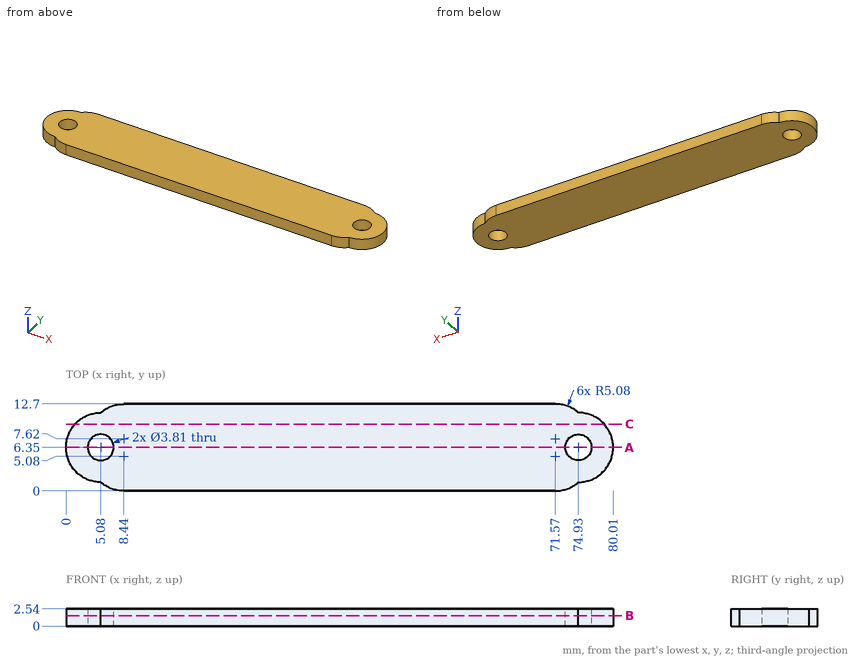
Here's the drawing with two shaded views (mm, measured from the low corner). I have some questions. Coordinates: 2 decimals unless noted, no trailing zeros. Order: outer loops, then holes, each group sorted by start corner. A loop starts at its lowest first (then second) coordinate and runs counter-clockwise, first axis right, second up. Notation, with made-up numbers: (-29.75, 80.5) - (27.25, 80.5) arc R15 cw to (27.25, 94.5) - close; hole circle Ø4 at (-19.5, -19.75). An arc over 180 degrees is marked (long way). Use CSV: the item, a comma, the result in double quotes. Start each with the question number.
1. Suppose I cut it at A-A on y = 6.35. List the corners of the cut face in (x, z) for me (3 decimals), then the cut area to 3 significant figures.
2. I'm going to push flat-ended pins straight in: pin 1 (1 mm diameter, centred on y = 9, z = 1.5, fed in from +X); pin 2 (2.5 mm diameter, centred on x = 74.93, y = 6.35, fed in from +Z). Where does each tip first touch, or does it pass through?
3. Suppose I cut it at C-C on y = 9.75. List the corners of the cut face in (x, z) for me.
4. Please list where these lines run through material, in increasing order: line 1 (Y direction, x = 5.08, z = 1.25) (1 decimal); line 2 (X direction, y = 8, z = 1.45) (1 decimal); line 3 (Y direction, x = 76.5, z = 0.4). Write a range as from..to.
5. Suppose I cut it at B-B on z = 1.55. List the corners of the cut face in (x, y) for me (3 decimals), then the cut area to 3 significant figures.
Output:
1,outline,"(0, 0) - (3.175, 0) - (3.175, 2.54) - (0, 2.54) - close; (6.985, 0) - (73.025, 0) - (73.025, 2.54) - (6.985, 2.54) - close; (76.835, 0) - (80.01, 0) - (80.01, 2.54) - (76.835, 2.54) - close"
1,area,"184 mm2"
2,pin 1,"stops at x = 79.53"
2,pin 2,"passes through"
3,outline,"(1.31, 0) - (78.7, 0) - (78.7, 2.54) - (1.31, 2.54) - close"
4,line 1,"y = 1.3..4.4, 8.3..11.4"
4,line 2,"x = 0.3..4.1, 6..74, 75.9..79.7"
4,line 3,"y = 1.52..5.27, 7.43..11.18"
5,outline,"(5.08, 1.27) arc R5.08 ccw to (8.44, 0) - (71.57, 0) arc R5.08 ccw to (74.93, 1.27) arc R5.08 ccw to (74.93, 11.43) arc R5.08 ccw to (71.57, 12.7) - (8.44, 12.7) arc R5.08 ccw to (5.08, 11.43) arc R5.08 ccw to start; hole circle Ø3.81 at (5.08, 6.35); hole circle Ø3.81 at (74.93, 6.35)"
5,area,"940 mm2"
